```python
from build123d import *

# Parameters (mm, degrees)
ESQUISSE1_R      = 3
EXTRUSION1_DEPTH = 16
ESQUISSE2_R      = 1.2
EXTRUSION2_DEPTH = 5
EXTRUSION3_START = 5.5
ESQUISSE3_R      = 1.2
EXTRUSION3_DEPTH = 5.5


with BuildPart() as part:
    # Esquisse1 → Extrusion1 (new body)
    with BuildSketch(Plane.XY):
        Circle(ESQUISSE1_R)
    extrude(amount=EXTRUSION1_DEPTH)

    # Esquisse2 → Extrusion2 (add)
    with BuildSketch(Plane.XY.offset(16)):
        Circle(ESQUISSE2_R)
    extrude(amount=EXTRUSION2_DEPTH)

    # Esquisse3 → Extrusion3 (add)
    with BuildSketch(Plane(origin=(0, 0, 0), x_dir=(-1, 0, 0), z_dir=(0, 0, -1)).offset(EXTRUSION3_START)):
        with Locations(Location((0, 0, 0), (0, 0, 180))):
            Circle(ESQUISSE3_R)
    extrude(amount=-EXTRUSION3_DEPTH)

    # Esquisse4 → Révolution1 (revolve)
    with BuildSketch(Plane(origin=(0, 0, 0), x_dir=(1, 0, 0), z_dir=(0, 1, 0))):
        Polygon((1.2, 5.5), (3, 1), (0, 1), (0, 5.5), align=None)
        Polygon((0, -21), (1.2, -21), (3, -17), (0, -17), align=None)
    revolve(axis=Axis((0, 0, 16), (0, 0, -1)))


solid = part.part
```
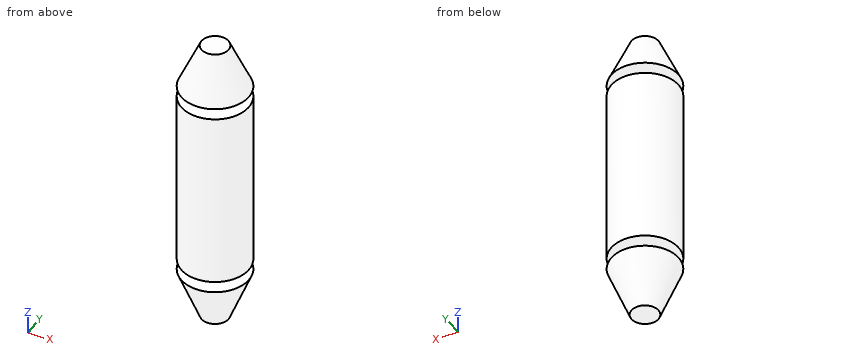
Input: part model. Units: mm. Frame: model coordinates. Round coordinates to 2 decimals unless told otherwise and drop trailing zeros. Loops run counter-clockwise (first coordinate to the right, second up) from the corner with the lowest first, then second, coordinate; pieces in that order, holes last. Notation, with made-up numbers: (73.25, 52) -> (126.25, 52) arc R28 cw to (126.25, 79) -> close; hole circle Ø1 at (5, 70.5). An arc over 180 degrees is marked (long way). Write each question's results on one line, items separated by ' | '.
1. Section D-D (y = -1.65). State how many separate pieces and enclosed holes the cut face has, and give its area (3 significant figures).
Geometry results:
separate pieces: 3 | enclosed holes: 0 | area: 100 mm2
2. Section A-A (x = 0). Return loops of the section in (y, z).
Geometry results:
outline: (-3, -1) -> (-1.2, -5.5) -> (1.2, -5.5) -> (3, -1) -> (1.2, -1) -> (1.2, 0) -> (3, 0) -> (3, 16) -> (1.2, 16) -> (1.2, 17) -> (3, 17) -> (1.2, 21) -> (-1.2, 21) -> (-3, 17) -> (-1.2, 17) -> (-1.2, 16) -> (-3, 16) -> (-3, 0) -> (-1.2, 0) -> (-1.2, -1) -> close
3. First-contact query: P1, Ø2, axis at x = 2, y = -2.5, coming from the +Z side. Flat tip, straight axial feed; report the tip coordinate or a pass-through.
Geometry results:
P1: z = 18.77
4. Section C-C (z = 7.5). Return loops of the section in (x, y), and give its area (3 significant figures).
Geometry results:
outline: circle Ø6 at (0, 0) | area: 28.3 mm2
5. Ray query, line 1 (Z direction, x = -0.5, y = 2.05); line 2 (Z direction, x = -0.4, y = 2.6); line 3 (X direction, y = 1.75, z = 1). Return the intervals inside material, ascending. Write a range as from..to.
Geometry results:
line 1: -3.22..-1, 0..16, 17..18.98 | line 2: -1.92..-1, 0..16, 17..17.82 | line 3: -2.44..2.44
